```python
from build123d import *

# Parameters (mm, degrees)
F0_W     = 44.637802
F0_H     = 44.637802
F0_R     = 2.15265
F0_R_2   = 2.285606
F0_R_3   = 7.9629
F1_DEPTH = 3.2512
F2_R     = 4.7625


with BuildPart() as f1:
    # F0 (on Top) → F1 (new body)
    with BuildSketch(Plane.XY):
        Rectangle(F0_W, F0_H)
        with Locations((-17.556401, -17.556401)):
            Circle(F0_R, mode=Mode.SUBTRACT)
        with Locations((-8.980259, -8.980259)):
            Circle(F0_R_2, mode=Mode.SUBTRACT)
        with Locations((17.556401, -17.556401)):
            Circle(F0_R, mode=Mode.SUBTRACT)
        with Locations((8.980259, -8.980259)):
            Circle(F0_R_2, mode=Mode.SUBTRACT)
        Circle(F0_R_3, mode=Mode.SUBTRACT)
        with Locations((-8.980259, 8.980259)):
            Circle(F0_R_2, mode=Mode.SUBTRACT)
        with Locations((-17.556401, 17.556401)):
            Circle(F0_R, mode=Mode.SUBTRACT)
        with Locations((8.980259, 8.980259)):
            Circle(F0_R_2, mode=Mode.SUBTRACT)
        with Locations((17.556401, 17.556401)):
            Circle(F0_R, mode=Mode.SUBTRACT)
    extrude(amount=F1_DEPTH)

    # F2
    f2_edges = [f1.edges().sort_by_distance(p)[0] for p in [
        (-22.318901, -22.318901, 1.6256),
        (22.318901, -22.318901, 1.6256),
        (22.318901, 22.318901, 1.6256),
        (-22.318901, 22.318901, 1.6256),
    ]]
    fillet(f2_edges, radius=F2_R)


solid = f1.part
```
CAD build for the part. Positions are in the model's coordinates, mm. Coordinates: 2 decimals unless noted, no trailing zeros. Order: outer loops, then holes, each group sorted by start corner. A loop starts at its lowest first (then second) coordinate and runs counter-clockwise, first axis right, second up. Notation, with made-up numbers: (22, -35.75) -> (26, -35.75) arc R7 cw to (26, -22.75) -> close; hole circle Ø8 at (21.25, 3.25). An arc over 180 degrees is marked (long way). Use one line per item in the form item = value. Start each with the question number.
1) Drill centre lines: L1, parallel to X at y = 17.5, z = 2.65; L2, parallel to Y at x = 8.5, z = 2.75; L3, parallel to X at y = 10, z = 1.25. Where is each one in solid material? Low to high. Write a range as [from, to].
2) Pull direction Y, two halves, no side cores. Call faces 1 (the cylindrical face through (20.89, 20.96, 1.65)), 2 (the cylindrical face through (20.89, -20.96, 1.65)), 3 (the cylindrical face through (-15.503, -16.91, 1.603)): +Y half, -Y half, draft (parallel to the pull), parting line (faces both ways), or undercut.
3) Band-saw the part on A-A on x = 0. Give the cut face in (y, z).
4) Band-saw the part on C-C on z = 1.2. State how many separate pieces and enclosed holes the cut face has, then the cut area to 3 significant figures.
5) Band-saw the part on D-D on y = 16. Give the cut face in (x, z).
Entries:
q1.L1 = [-22.32, -19.71], [-15.4, 15.4], [19.71, 22.32]
q1.L2 = [-22.32, -11.21], [-6.75, 6.75], [11.21, 22.32]
q1.L3 = [-22.32, -11.03], [-6.93, 6.93], [11.03, 22.32]
q2.face_1 = +Y half
q2.face_2 = -Y half
q2.face_3 = undercut
q3.outline = (-22.32, 0) -> (-7.96, 0) -> (-7.96, 3.25) -> (-22.32, 3.25) -> close; (7.96, 0) -> (22.32, 0) -> (22.32, 3.25) -> (7.96, 3.25) -> close
q4.separate_pieces = 1
q4.enclosed_holes = 9
q4.area = 1,650 mm2
q5.outline = (-22.32, 0) -> (-19.04, 0) -> (-19.04, 3.25) -> (-22.32, 3.25) -> close; (-16.07, 0) -> (16.07, 0) -> (16.07, 3.25) -> (-16.07, 3.25) -> close; (19.04, 0) -> (22.32, 0) -> (22.32, 3.25) -> (19.04, 3.25) -> close
